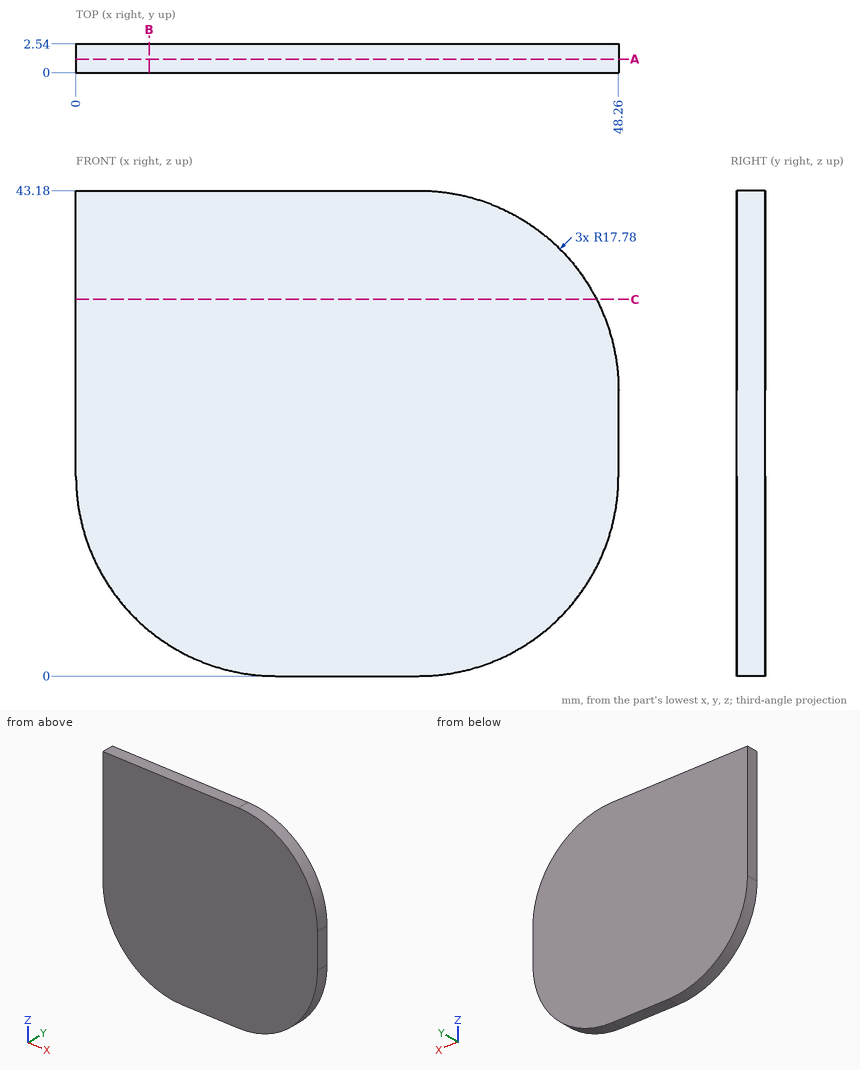
The drawing under review shows one solid part. Ordinate dimensions are in mm from its lowest x, y, z. Give positions to 0.01 mm unless a question says otherwise; leave off trailing zeros. Write each loop counter-clockwise with the first axis right and the second up, starting at its lowest first coordinate (ties: lowest second). Pieces come first, ordered by that corner, then holes. Notation, with made-up numbers: (41, -18.5) -> (77, -18.5) arc R13 cw to (77, -14.5) -> close; hole circle Ø6 at (79.5, 14). An arc over 180 degrees is marked (long way). Put each result on its own line as item: value.
(1) We need section A-A, the plane y = 1.2. Give the boundary of the cut face in (x, z).
Results are:
outline: (0, 17.78) arc R17.78 ccw to (17.78, 0) -> (30.48, 0) arc R17.78 ccw to (48.26, 17.78) -> (48.26, 25.4) arc R17.78 ccw to (30.48, 43.18) -> (0, 43.18) -> close
(2) For pin 1 Ø1.5 at (x, y) = (37, 1) entering from +Z, flat-tipped, find the tip position at first contact; note if it passes through.
Results are:
pin 1: z = 42.22
(3) We need section B-B, the plane x = 6.5. Give the boundary of the cut face in (y, z), and give its area (3 significant figures).
Results are:
outline: (0, 4.04) -> (2.54, 4.04) -> (2.54, 43.18) -> (0, 43.18) -> close
area: 99.4 mm²
(4) To check wall thickness, follow probe 1 along X at (y, z) = (0.3, 26); probe 2 along Z at (x, y) = (36.5, 1.15); probe 3 along X at (y, z) = (0.7, 12.5). State the ranges of each line that lie inside material, in increasing order. Write a range as from..to.
Results are:
probe 1: 0..48.25
probe 2: 1.05..42.13
probe 3: 0.8..47.46
(5) We need section C-C, the plane z = 33.5. Give the boundary of the cut face in (x, y).
Results are:
outline: (0, 0) -> (46.31, 0) -> (46.31, 2.54) -> (0, 2.54) -> close
